Autodesk Inventor part; units mm, degrees
ref_plane "YZ Plane" through (0, 0, 0) normal (1, 0, 0) x (0, 1, 0)
ref_plane "XY Plane" through (0, 0, 0) normal (0, 0, 1) x (1, 0, 0)
sketch "Sketch1" plane through (0, 0, 0) normal (0, 0, 1) x (1, 0, 0)
  line L0 (-6.5, 5.5) -> (6.5, 5.5)
  line L1 (6.5, 5.5) -> (6.5, -5.5)
  line L2 (6.5, -5.5) -> (-6.5, -5.5)
  line L3 (-6.5, -5.5) -> (-6.5, 5.5)
  point P0 (0, 0)
  dimension "d0" = 13
  dimension "d1" = 11
  dimension "d2" = 6.5
  dimension "d3" = 5.5
extrude "Extrusion1" add sketch "Sketch1" against normal blind 200
sketch "Sketch2" plane through (0, 0, 0) normal (0, 0, 1) x (1, 0, 0)
  line L0 (-6.5, 5.5) -> (6.5, 5.5)
  line L1 (-6.5, -5.5) -> (-6.5, 5.5)
  line L2 (6.5, -5.5) -> (-6.5, -5.5)
  line L3 (6.5, 5.5) -> (6.5, -5.5)
  line L4 (-6.5, 4.5) -> (-4.2125, 4.5)
  line L5 (-4.2125, 4.5) -> (-4.2125, -0.1875)
  line L6 (-4.2125, -0.1875) -> (-4, -0.4)
  line L7 (-4, -0.4) -> (-4, -5.5)
  line L8 (0, 7.7) -> (0, -7.7)
  line L9 (-6.5, 4.5) -> (-6.5, -5.5)
  line L10 (-6.5, -5.5) -> (-4, -5.5)
  dimension "d6" = 1
  dimension "d7" = 8.425
  dimension "d8" = 8
  dimension "d9" = 135
  dimension "d10" = 5.1
extrude "Extrusion2" cut sketch "Sketch2" against normal through all contours L4 L5 L6 L7 L2 L1
fillet "Fillet1" radius 1 1 edges at (-4.2125, 4.5, -100)
fillet "Fillet1" radius 1.1 1 edges at (-4, -5.5, -100)
mirror "Mirror1" about plane through (0, 0, 0) normal (1, 0, 0) of "Extrusion2", "Fillet1"
sketch "Sketch3" plane through (0, 0, 0) normal (0, 0, 1) x (1, 0, 0)
  line L0 (-6.5, 5.5) -> (6.5, 5.5)
  line L1 (-4.2125, 3.5) -> (-4.2125, -0.1875)
  line L2 (-4.2125, -0.1875) -> (-4, -0.4)
  line L3 (-4, -0.4) -> (-4, -4.4)
  line L4 (2.9, -5.5) -> (-2.9, -5.5)
  arc A0 (-3.05, 5.1) -> (-3.05, 5.5) centre (-3.05, 5.3) ccw
  line L5 (-3.1625, 0.2474) -> (-2.95, 0.0349)
  line L6 (-2.95, 0.0349) -> (-2.95, -4.46)
  line L7 (-2.95, -4.46) -> (-0.9867, -4.46)
  line L8 (0, 7.7) -> (0, -7.7)
  line L9 (-3.1625, 0.2474) -> (-3.1625, 5.1)
  line L10 (-3.05, 5.1) -> (-3.1625, 5.1)
  line L11 (-0.775, 1.6018) -> (-0.9867, -4.46)
  line L12 (0, 1.5) -> (0, -5.5)
  arc A1 (-0.775, 1.6018) -> (0, 1.5) centre (0, 4.5) ccw
  line L13 (0, 1.5) -> (0, 5.5)
  line L14 (0, 5.5) -> (-3.05, 5.5)
  dimension "d15" = 0.4
  dimension "d16" = 1
  dimension "d18" = 5.7
  dimension "d19" = 1.05
  dimension "d20" = 1.05
  dimension "d21" = 1.05
  dimension "d22" = 92
  dimension "d23" = 1.04
  dimension "d24" = 1.55
  dimension "d25" = 3
extrude "Extrusion3" cut sketch "Sketch3" against normal through all
mirror "Mirror2" about plane through (0, 0, 0) normal (1, 0, 0) of "Extrusion3"
fillet "Fillet2" radius 0.4 4 edges at (-2.95, -4.46, -100) (-0.9867, -4.46, -100) (0.9867, -4.46, -100) (2.95, -4.46, -100)
ref_plane "Side1" through (-6.5, 4.5, 0) normal (0, -1, 0) x (1, 0, 0)
ref_plane "T-Slot1" through (0, 5.5, 0) normal (1, 0, 0) x (0, 0, -1)
ref_plane "Side3" through (-6.5, 5.5, 0) normal (0, 1, 0) x (-1, 0, 0)
ref_plane "Side2" through (6.5, 5.5, 0) normal (1, 0, 0) x (0, 1, 0)
ref_plane "Piano di lavoro5" through (0, 1.5, 0) normal (0, 1, 0) x (-1, 0, 0)
equation "\"d4\" = Ex_Length"
equation "\"Ex_Length\" = 200"
properties part number "13-106" material "Alluminio - 6061"
Work out the finished part from the listing and answer in its coordinate system (mm). A direction names the side the tool comes from. Coordinates: 2 decimals unless noted, no trailing zeros.
1) For faces 1 (the flat face through (3.162, 3, -99)), 2 (the flat face through (-4.212, 2, -99)), 3 (the flat face through (4, -2, -99)), determine the directions among +Z, -Z, +X, -X, +Y, -Y from which every point of the face is accessible in a straight line to the end or side of a thin tool.
Results:
face 1: +Z, -Z
face 2: +Z, -Z, -X, -Y
face 3: +Z, -Z, +X, -Y
2) Flat-ended cylindrical pins translate along their axes: pin 1 (3 mm diameter, centred on y = 1.5, z = -81, fed in from -X); pin 2 (1 mm diameter, centred on x = -6, z = -61.5, fed in from -Y); pin 3 (2 mm diameter, centred on y = -1.5, z = -105.5, fed in from +X); pin 4 (6 mm diameter, centred on x = 2.5, z = -163.5, fed in from +Y). Find the tip coordinate at first contact, or state that the pin passes through.
Results:
pin 1: stops at x = -4.21
pin 2: stops at y = 4.5
pin 3: stops at x = 4
pin 4: stops at y = 5.5
3) Consider probe 1 along X at (y, z) = (-3.25, -68); probe 2 along X at (y, z) = (-3.5, -172); probe 3 along X at (y, z) = (2.5, -158.5). Determine where each line is inside the solid, lowest interval first.
Results:
probe 1: x = -4 to -2.95, -0.94 to 0.94, 2.95 to 4
probe 2: x = -4 to -2.95, -0.95 to 0.95, 2.95 to 4
probe 3: x = -4.21 to -3.16, 3.16 to 4.21
